The drawing under review shows one solid part. Ordinate dimensions are in mm from its lowest x, y, z. Give positions to 0.01 mm unless a question says otherwise; leave off trailing zeros. Write each loop counter-clockwise with the first axis right and the second up, starting at its lowest first coordinate (ties: lowest second). Pieces come first, ordered by that corner, then holes. Notation, with made-up numbers: M 29.25,25.25 L 50.25,25.25 A24 cw 50.25,49.25 Z; hole C -11,66 d10. An arc over 180 degrees is marked long. Write item = value, one per line. Start each with the question number.
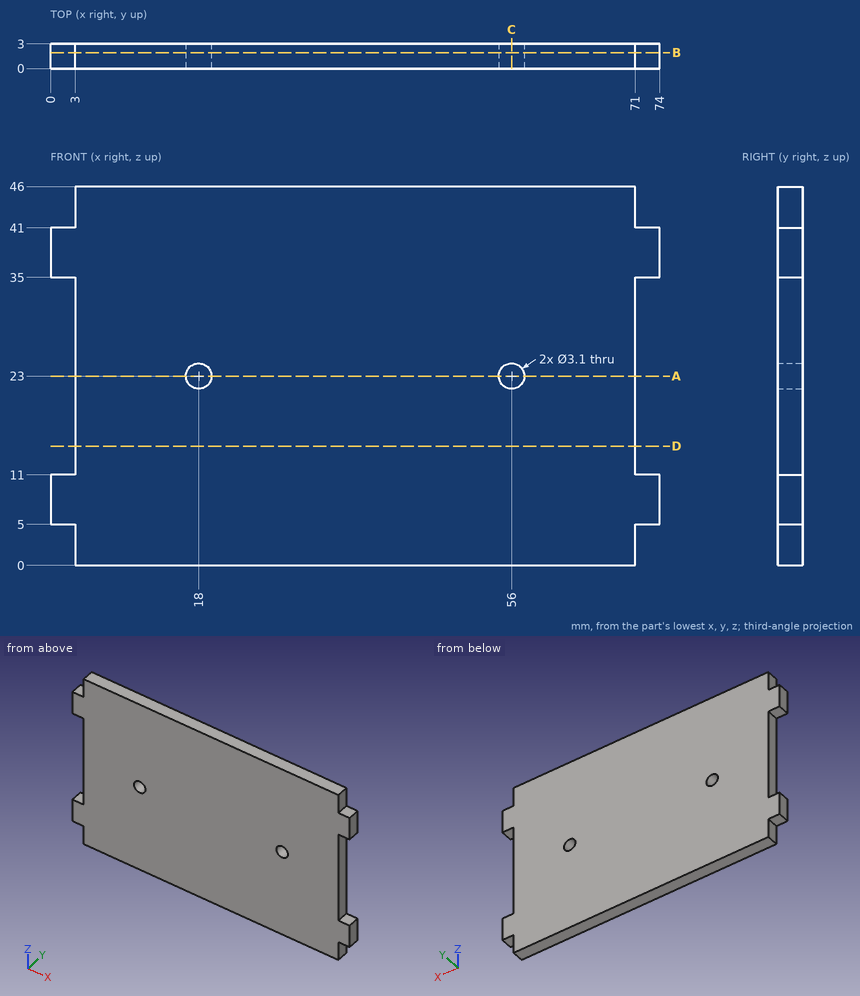
Item 1: To check wall thickness, follow probe 1 along X at (y, z) = (1.9, 23); probe 2 along Z at (x, y) = (18, 1.65); probe 3 along X at (y, z) = (0.2, 20). State the ranges of each line that lie inside material, in increasing order. Write a range as [from, to].
Item 2: We need section D-D, the plane z = 14.5. Write out the cut boundary in (x, y).
Item 3: We need section C-C, the plane x = 56. Write out the cut boundary in (y, z), and give its area (3 significant figures).
Item 4: We need section B-B, the plane y = 1.95. Write out the cut boundary in (x, z), and give its area (3 significant figures).
Item 5: We need section A-A, the plane z = 23. Write out the cut boundary in (x, y).
Item 6: Clearance check with flat-ended pins moving along their axes: P1, Ø0.9, axis at y = 2, z = 2.5, coming from the +X side; P2, Ø1.5, axis at y = 1.5, z = 44, coming from the -X side; P3, Ø1.5, axis at x = 2, y = 1, coming from the -Z side. State where each tip first meets the part, or that it passes through.
Worked out:
q1.probe_1 = [3, 16.45], [19.55, 54.45], [57.55, 71]
q1.probe_2 = [0, 21.45], [24.55, 46]
q1.probe_3 = [3, 71]
q2.outline = M 3,0 L 71,0 L 71,3 L 3,3 Z
q3.outline = M 0,0 L 3,0 L 3,21.45 L 0,21.45 Z; M 0,24.55 L 3,24.55 L 3,46 L 0,46 Z
q3.area = 129 mm²
q4.outline = M 0,5 L 3,5 L 3,0 L 71,0 L 71,5 L 74,5 L 74,11 L 71,11 L 71,35 L 74,35 L 74,41 L 71,41 L 71,46 L 3,46 L 3,41 L 0,41 L 0,35 L 3,35 L 3,11 L 0,11 Z; hole C 18,23 d3.1; hole C 56,23 d3.1
q4.area = 3,180 mm²
q5.outline = M 3,0 L 16.45,0 L 16.45,3 L 3,3 Z; M 19.55,0 L 54.45,0 L 54.45,3 L 19.55,3 Z; M 57.55,0 L 71,0 L 71,3 L 57.55,3 Z
q6.P1 = 71
q6.P2 = 3
q6.P3 = 5
